Could you check a few things on this model? Use its own coordinates, in mm. Face numbers are marked on the shaded views. A direction names the side the tool comes from. Give positions to 0.01 mm unless a question says otherwise; leave off trailing zeros. Order: outer loops, then holes, each group sorted by start corner. A loop starts at its lowest first (then second) coordinate and runs counter-clockwise, first axis right, second up.
(1) Imagine slicing it at B-B, the plane z = -14.25. Write out the boundary of the cut face in (x, y), then the cut area to 3 significant figures.
(2) Imagine slicing it at C-C, the plane x = 2.5. Write out the boundary of the cut face in (y, z), then the cut area to 3 significant figures.
(3) On a 3-axis mill with a long thin cutter (end or side, diameter ignored), from which of +Z, -Z, +X, -X, +Y, -Y can I reach the whole of each face in a straight line? I mean the marked faces 5, 6 and 7. Say none if no direction works.
(4) Imagine slicing it at D-D, the plane z = -4.75. Write out the boundary of the cut face in (x, y), then the cut area to 3 significant figures.
(5) If we mould it in two halves opening along X, with no side actions, what happens to the marked faces 1, 2, 3 and 4? For each: released by +X, released by -X, zero draft, split by the parting line, or undercut.
(6) Imagine slicing it at A-A, the plane y = -3.75. Write out the boundary of the cut face in (x, z), then the cut area to 3 significant figures.
(7) If I drill on probe 1 along Y at (x, z) = (-0.75, -0.75); probe 2 along Z at (x, y) = (-2, -4.75); probe 3 along Y at (x, z) = (-2.25, -14.25), over which ranges is the centre line in solid material (lowest first)?
(8) Will these pins go through, and if not, where does the flat tip stop? pin 1 (1.9 mm diameter, centred on x = -4, y = -4, fed in from +Z); pin 2 (1.1 mm diameter, centred on x = -3.5, y = -4, fed in from -Z); pin 3 (1 mm diameter, centred on x = 10, y = -4, fed in from -Z).
from build123d import *

# Parameters (mm, degrees)
SKETCH1_W               = 20
SKETCH1_H               = 20
BOSS_EXTRUDE1_DEPTH     = 7.5
SKETCH6_W               = 20
SKETCH6_H               = 20
CUT_EXTRUDE1_DEPTH      = 8
SKETCH8_R               = 1
BOSS_EXTRUDE3_DEPTH     = 5
CUT_EXTRUDE2_DEPTH      = 0.5
CUT_EXTRUDE2_DEPTH_BACK = 0.5
SKETCH9_W               = 20
SKETCH9_H               = 7
CUT_EXTRUDE3_DEPTH      = 0.5
CUT_EXTRUDE3_DEPTH_BACK = 0.5
SKETCH10_W              = 20
SKETCH10_H              = 7


with BuildPart() as part:
    # Sketch1 → Boss-Extrude1 (new body)
    with BuildSketch(Plane(origin=(0, 0, 0), x_dir=(1, 0, 0), z_dir=(0, 1, 0))):
        with Locations((4.807692308, 6.842948718)):
            Rectangle(SKETCH1_W, SKETCH1_H)
    extrude(amount=BOSS_EXTRUDE1_DEPTH)

    # Sketch3 → Cut-Revolve3 (revolve, cut)
    with BuildSketch(Plane.XY.offset(-6.842948718)):
        with BuildLine():
            ThreePointArc((4.807692308, -13), (12.807692308, -5), (4.807692308, 3))
            Line((4.807692308, 3), (4.807692308, -13))
        make_face()
    revolve(axis=Axis((4.807692308, 5, -6.842948718), (0, -1, 0)), mode=Mode.SUBTRACT)

    # Sketch5 → Revolve7 (revolve)
    with BuildSketch(Plane.XY.offset(-6.842948718)):
        with BuildLine():
            ThreePointArc((4.807692308, -13), (12.807692308, -5), (4.807692308, 3))
            Line((4.807692308, 3), (4.807692308, 5))
            ThreePointArc((4.807692308, 5), (14.807692308, -5), (4.807692308, -15))
            Line((4.807692308, -15), (4.807692308, -13))
        make_face()
    revolve(axis=Axis((4.807692308, 5, -6.842948718), (0, -1, 0)))

    # Sketch6 → Cut-Extrude1 (cut)
    with BuildSketch(Plane(origin=(0, -15, 0), x_dir=(-1, 0, 0), z_dir=(0, -1, 0))):
        with Locations((-4.807692308, 6.842948718)):
            Rectangle(SKETCH6_W, SKETCH6_H)
    extrude(amount=-CUT_EXTRUDE1_DEPTH, mode=Mode.SUBTRACT)

    # Sketch8 → Boss-Extrude3 (add)
    with BuildSketch(Plane(origin=(0, 7.5, 0), x_dir=(1, 0, 0), z_dir=(0, 1, 0))):
        with Locations(Location((-2.192307692, -0.157051282, 0), (0, 0, 90))):
            Circle(SKETCH8_R)
        with Locations(Location((-2.192307692, 13.842948718, 0), (0, 0, 90))):
            Circle(SKETCH8_R)
        with Locations(Location((11.807692308, -0.157051282, 0), (0, 0, 90))):
            Circle(SKETCH8_R)
        with Locations(Location((11.807692308, 13.842948718, 0), (0, 0, 90))):
            Circle(SKETCH8_R)
    extrude(amount=BOSS_EXTRUDE3_DEPTH)

    # Sketch9 → Cut-Extrude2 (cut, two sides: drawn at the far end of the back side and taken through both)
    with BuildSketch(Plane.XY.offset(-6.842948718).offset(-CUT_EXTRUDE2_DEPTH_BACK)):
        with Locations((4.807692308, -3.5)):
            Rectangle(SKETCH9_W, SKETCH9_H)
    extrude(amount=CUT_EXTRUDE2_DEPTH + CUT_EXTRUDE2_DEPTH_BACK, mode=Mode.SUBTRACT)


with BuildPart() as cut_extrude2_kept_piece:
    # of the separate pieces the step leaves, the one the design keeps (cut_extrude2_pieces_kept)
    add(part.part.solids().sort_by_distance((-5.192307692, 0, 3.157051282))[0])

    # Sketch10 → Cut-Extrude3 (cut, two sides: drawn at the far end of the back side and taken through both)
    with BuildSketch(Plane.ZY.offset(-4.807692308).offset(-CUT_EXTRUDE3_DEPTH_BACK)):
        with Locations((-6.842948718, -3.5)):
            Rectangle(SKETCH10_W, SKETCH10_H)
    extrude(amount=CUT_EXTRUDE3_DEPTH + CUT_EXTRUDE3_DEPTH_BACK, mode=Mode.SUBTRACT)


with BuildPart() as cut_extrude3_kept_piece:
    # of the separate pieces the step leaves, the one the design keeps (cut_extrude3_pieces_kept)
    add(cut_extrude2_kept_piece.part.solids().sort_by_distance((-5.192307692, 0, 3.157051282))[0])


solid = cut_extrude3_kept_piece.part
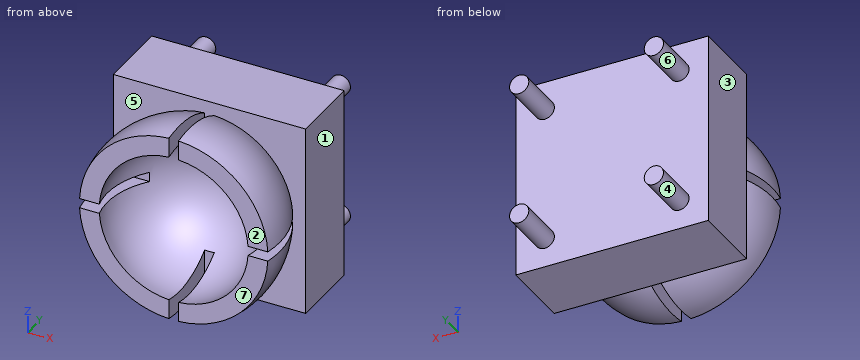
Answer block:
1. outline: (-5.19, 0) - (0.32, 0) arc R6.72 ccw to (-1.61, -7) - (2.54, -7) arc R3.02 cw to (4.31, -2.02) - (4.31, 0) - (5.31, 0) - (5.31, -2.02) arc R3.02 cw to (7.07, -7) - (11.22, -7) arc R6.72 ccw to (9.29, 0) - (14.81, 0) - (14.81, 7.5) - (12.72, 7.5) - (12.72, 12.5) - (10.89, 12.5) - (10.89, 7.5) - (-1.28, 7.5) - (-1.28, 12.5) - (-3.11, 12.5) - (-3.11, 7.5) - (-5.19, 7.5) - close
1. area: 228 mm2
2. outline: (-7, -16.37) arc R9.73 ccw to (0, -15.19) - (0, -16.84) - (7.5, -16.84) - (7.5, 3.16) - (0, 3.16) - (0, 1.5) arc R9.73 ccw to (-7, 2.68) - (-7, 0.55) arc R7.66 cw (long way) to (-7, -14.24) - close
2. area: 159 mm2
3. face 5: none
3. face 6: +Y
3. face 7: +Z, -Z, +X, -X, -Y
4. outline: (-5.19, 0) - (-3.6, 0) arc R9.78 ccw to (-4.76, -7) - (-2.65, -7) arc R7.72 cw (long way) to (12.27, -7) - (14.38, -7) arc R9.78 ccw to (13.21, 0) - (14.81, 0) - (14.81, 7.5) - (-5.19, 7.5) - close
4. area: 158 mm2
5. face 1: released by +X
5. face 2: zero draft
5. face 3: released by -X
5. face 4: undercut
6. outline: (-5.1, -7.34) arc R9.92 ccw to (4.31, -16.75) - (4.31, -14.73) arc R7.9 cw to (-3.08, -7.34) - close; (-5.1, -6.34) - (-3.08, -6.34) arc R7.9 cw to (4.31, 1.04) - (4.31, 3.07) arc R9.92 ccw to start; (5.31, -16.75) arc R9.92 ccw to (14.72, -7.34) - (12.69, -7.34) arc R7.9 cw to (5.31, -14.73) - close; (5.31, 1.04) arc R7.9 cw to (12.69, -6.34) - (14.72, -6.34) arc R9.92 ccw to (5.31, 3.07) - close
6. area: 105 mm2
7. probe 1: y = -7 to 7.5
7. probe 2: z = -14.16 to -11.04, -2.65 to 0.48
7. probe 3: y = 0 to 12.5
8. pin 1: stops at z = -0.73
8. pin 2: stops at z = -13.08
8. pin 3: stops at z = -15.62
